Input: part model. Units: mm. Frame: model coordinates. A direction names the side the tool comes from. Coordinates: 2 decimals unless noted, no trailing zeros. Order: outer loops, then holes, each group sorted by start corner. A loop starts at its lowest first (then second) coordinate and runs counter-clockwise, first axis right, second up. Notation, with made-up numbers: (63.5, -39.75) -> (99.5, -39.75) arc R21 ccw to (99.5, -6.75) -> close; hole circle Ø9 at (75, -13). An arc over 180 degrees is marked (long way). One line per item, written item: value. Start each with the question number.
from build123d import *

# Parameters (mm, degrees)
M6_TAPPED_HOLE1_D = 5


with BuildPart() as part:
    # Sketch1 → Revolve1 (revolve)
    with BuildSketch(Plane.XY, mode=Mode.PRIVATE) as revolve1_sk:
        Polygon((20, -121.747729768), (20, 61.139021578), (66.961524227, 88.252270232), (83.301270189, 88.252270232), (83.301270189, 83.252270232), (68.301270189, 83.252270232), (25, 58.252270232), (25, -111.747729768), (30, -111.747729768), (30, -121.747729768), (25, -121.747729768), align=None)
    revolve(revolve1_sk.sketch.rotate(Axis((0, 0, 0), (0, 1, 0)), 90), axis=Axis((0, 0, 0), (0, 1, 0)))

    # M6 Tapped Hole1 (through all)
    with Locations(Plane(origin=(-56, 88.252270232, -56), x_dir=(0, 0, 1), z_dir=(0, 1, 0))):
        with Locations((0, 0), (0, 112), (112, 0), (112, 112)):
            Hole(M6_TAPPED_HOLE1_D / 2)


solid = part.part
1) Section query D-D, the plane y = 66.5. Return the cut outline in (x, z).
2) Section query B-B, the plane z = 0. Return the cut outline in (x, y), plus the area to 3 significant figures.
3) Section query A-A, the plane x = 0. Return the cut outline in (y, z), plus the area to 3 significant figures.
4) Ray query, line 1 along X through (y, z) = (-18, 0); line 2 along Y through (x, z) = (-5, 76); line 3 along X through (y, z) = (15, 10.5). Return the intervals inside material, ascending. Write a range as from..to.
5) Pin query (flat end, axial travel): pin 1 Ø4 at (x, z) = (-56, 56) entering from -Y; pin 2 Ø4 at (x, z) = (-47, 20) entering from -Y; pin 3 Ø8 at (y, z) = (38, 5) entering from -X; pin 4 Ø6 at (x, z) = (56, -56) entering from -Y. Return the tip coordinate at first contact, or that it passes through.
6) Mould query, pull axis Z, two halves, no side actions, for faces 1 (the cylindrical face through (-25.296, -116.818, -16.128)), 2 (the conical face through (22.392, 62.835, 4.972)), 3 (the flat face through (-68, 88.252, 0)). Classes: +Z half, -Z half, draft (parallel to the pull), parting line (faces both ways), or undercut.
7) Section query C-C, the plane y = -18.5. Return the cut outline in (x, z), plus the area to 3 significant figures.
8) Access query for faces 4 (the flat face through (-68.3, 83.252, 6.6)), 5 (the cylindrical face through (-0.88, -29.02, 19.98)), 6 (the cylindrical face through (-7.509, -27.938, -23.846)). Directions: +Z, -Z, +X, -X, +Y, -Y. A direction counts if a zero-diameter tool reaches every point of the face in a straight line with its end or side. Return the directions, or none.
Entries:
1. outline: circle Ø78.57 at (0, 0); hole circle Ø58.57 at (0, 0)
2. outline: (-83.3, 83.25) -> (-68.3, 83.25) -> (-25, 58.25) -> (-25, -111.75) -> (-30, -111.75) -> (-30, -121.75) -> (-20, -121.75) -> (-20, 61.14) -> (-66.96, 88.25) -> (-83.3, 88.25) -> close; (20, -121.75) -> (30, -121.75) -> (30, -111.75) -> (25, -111.75) -> (25, 58.25) -> (68.3, 83.25) -> (83.3, 83.25) -> (83.3, 88.25) -> (66.96, 88.25) -> (20, 61.14) -> close
2. area: 2,590 mm2
3. outline: (-121.75, -30) -> (-111.75, -30) -> (-111.75, -25) -> (58.25, -25) -> (83.25, -68.3) -> (83.25, -83.3) -> (88.25, -83.3) -> (88.25, -66.96) -> (61.14, -20) -> (-121.75, -20) -> close; (-121.75, 20) -> (61.14, 20) -> (88.25, 66.96) -> (88.25, 83.3) -> (83.25, 83.3) -> (83.25, 68.3) -> (58.25, 25) -> (-111.75, 25) -> (-111.75, 30) -> (-121.75, 30) -> close
3. area: 2,590 mm2
4. line 1: x = -25..-20, 20..25
4. line 2: y = 83.25..88.25
4. line 3: x = -22.69..-17.02, 17.02..22.69
5. pin 1: passes through
5. pin 2: stops at y = 72.15
5. pin 3: stops at x = -24.98
5. pin 4: stops at y = 83.25
6. face 1: parting line
6. face 2: undercut
6. face 3: draft
7. outline: circle Ø50 at (0, 0); hole circle Ø40 at (0, 0)
7. area: 707 mm2
8. face 4: -Y
8. face 5: +Y, -Y
8. face 6: none
